Source: CAD feature listing. Evaluate the final solid. Frame: model axes, mm. A direction names the side the tool comes from. Coordinates: 2 decimals unless noted, no trailing zeros. Order: outer loops, then holes, each group sorted by start corner. A loop starts at its lowest first (then second) coordinate and runs counter-clockwise, first axis right, second up.
Item 1: Reachability of faces 4 (the flat face through (0, 0, 1.3)), 5 (the flat face through (1, 0, 1)) from +Z, -Z, +X, -X, +Y, -Y: full face, straight path, thin tool, end or side. Return the list, or none.
Item 2: Section C-C on x = 4.25. Return the cut outline in (y, z), then the cut area to 3 significant figures.
Item 3: Mould query, pull axis Z, two halves, no side actions, for faces 1 (the cylindrical face through (3.63, -1.5, -0.07)), 2 (the flat face through (6, 0, 0)), 3 (the flat face through (1, 0, -1)). Classes: released by +Z, released by -Z, zero draft, split by the parting line, or undercut.
Item 4: Section A-A on x = 0.75. Return the cut outline in (y, z).
Item 5: Section B-B on y = 0. Return the cut outline in (x, z), then the cut area to 3 significant figures.
Item 6: Ray query, line 1 (X direction, y = 1.95, z = 2); line 2 (X direction, y = 1.95, z = -0.8); line 3 (Z direction, x = 3.75, y = -0.2). Return the intervals inside material, ascending.
from build123d import *

# Parameters (mm, degrees)
CHANFREIN1_SIZE         = 0.5
ENL_V_MAT_EXTRU_1_DEPTH = 1.2


with BuildPart() as part:
    # Esquisse1 → Révolution1 (revolve)
    with BuildSketch(Plane.XY):
        Polygon((0, 0), (0, 3), (0.2, 3), (1.7, 1.5), (6, 1.5), (6, 0), align=None)
    revolve(axis=Axis((6, 0, 0), (-1, 0, 0)))

    # Chanfrein1
    chanfrein1_edges = [part.edges().sort_by_distance(p)[0] for p in [
        (6, -1.5, 0),
    ]]
    chamfer(chanfrein1_edges, length=CHANFREIN1_SIZE)

    # Esquisse2 → Enlèv. mat.-Extru.1 (cut)
    with BuildSketch(Plane.ZY):
        Polygon((0, 1.154700538), (-1, 0.577350269), (-1, -0.577350269), (0, -1.154700538), (1, -0.577350269), (1, 0.577350269), align=None)
    extrude(amount=-ENL_V_MAT_EXTRU_1_DEPTH, mode=Mode.SUBTRACT)


solid = part.part
Answer list:
1. face 4: +Z, -Z, -X, +Y, -Y
1. face 5: -X
2. outline: circle Ø3 at (0, 0)
2. area: 7.07 mm2
3. face 1: split by the parting line
3. face 2: zero draft
3. face 3: undercut
4. outline: circle Ø4.9 at (0, 0); hole (-1.15, 0) - (-0.58, -1) - (0.58, -1) - (1.15, 0) - (0.58, 1) - (-0.58, 1) - close
5. outline: (0, -3) - (0.2, -3) - (1.7, -1.5) - (5.5, -1.5) - (6, -1) - (6, 1) - (5.5, 1.5) - (1.7, 1.5) - (0.2, 3) - (0, 3) - (0, 1) - (1.2, 1) - (1.2, -1) - (0, -1) - close
5. area: 18.2 mm2
6. line 1: x = 0 to 0.41
6. line 2: x = 0 to 1.09
6. line 3: z = -1.49 to 1.49
